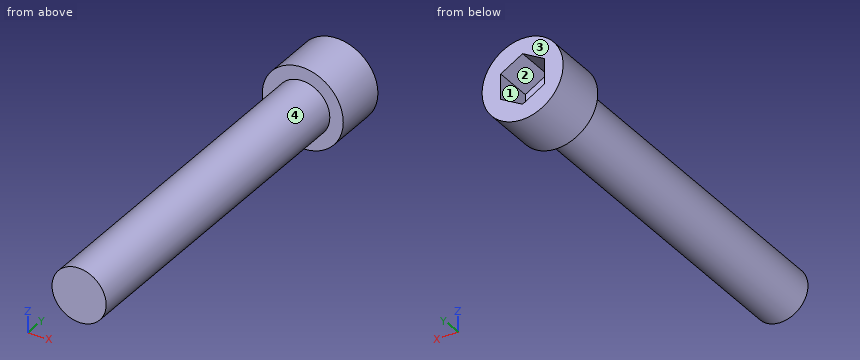
from build123d import *

# Parameters (mm, degrees)
SKETCH1_R           = 5.875
BOSS_EXTRUDE1_DEPTH = 7.75
CUT_EXTRUDE1_DEPTH  = 5.5
SKETCH3_R           = 3.925
BOSS_EXTRUDE2_DEPTH = 10
SKETCH4_R           = 3.925
BOSS_EXTRUDE3_DEPTH = 40


with BuildPart() as part:
    # Sketch1 → Boss-Extrude1 (new body)
    with BuildSketch(Plane(origin=(0, 0, 0), x_dir=(1, 0, 0), z_dir=(0, 1, 0))):
        Circle(SKETCH1_R)
    extrude(amount=BOSS_EXTRUDE1_DEPTH)

    # Sketch2 → Cut-Extrude1 (cut)
    with BuildSketch(Plane(origin=(0, 7.75, 0), x_dir=(1, 0, 0), z_dir=(0, 1, 0))):
        Polygon((0, 3.666174209), (-3.175, 1.833087105), (-3.175, -1.833087105), (0, -3.666174209), (3.175, -1.833087105), (3.175, 1.833087105), align=None)
    extrude(amount=-CUT_EXTRUDE1_DEPTH, mode=Mode.SUBTRACT)

    # Sketch3 → Boss-Extrude2 (add)
    with BuildSketch(Plane.XZ):
        Circle(SKETCH3_R)
    extrude(amount=BOSS_EXTRUDE2_DEPTH)

    # Sketch4 → Boss-Extrude3 (add)
    with BuildSketch(Plane.XZ.offset(10)):
        Circle(SKETCH4_R)
    extrude(amount=BOSS_EXTRUDE3_DEPTH)


solid = part.part
Check sheet for the modelled part. Datum: model origin and axes. Units: mm. Face numbers are marked on the shaded views. Give positions to 0.01 mm unless a question says otherwise; leave off trailing zeros. Loops run counter-clockwise (first coordinate to the right, second up) from the corner with the lowest first, then second, coordinate; pieces in that order, holes last. Notation, with made-up numbers: M -21.75,46 L 0.25,46 A30 cw 0.25,72 Z; hole C 44.25,37.5 d10. An arc over 180 degrees is marked long. Return JSON: item names as keys, results as strings. Group by question number.
1. Cross-section at C-C on y = -44. Record the boundary of the cut face in (x, z) (3 decimals).
2. Cross-section at B-B on x = 1.5. Record the boundary of the cut face in (y, z).
3. Thickness scan on L1, parallel to Y at x = -2.5, z = -4.5; L2, parallel to X at y = -5.5, z = -0.25; L3, parallel to Y at x = 2.5, z = 0.25. Record the ranges inside material, lowest first.
4. Mould release check, pull along Z, two halves, no side actions. Record for the marked faces 1, 2, 3 and 4: released by +Z, released by -Z, zero draft, split by the parting line, or undercut.
5. Cross-section at A-A on z = 0. Record the boundary of the cut face in (x, y) (3 decimals), plus the area to 3 significant figures.
6. Cross-section at D-D on z = -5. Record the boundary of the cut face in (x, y), plus the area to 3 significant figures.
7. Go/stop test with flat-tipped pins: pin 1 (5 mm diameter, centred on y = -19.5, z = -2.5, fed in from -X) (3 decimals); pin 2 (5 mm diameter, centred on x = 1.5, y = -29, fed in from -Z) (3 decimals); pin 3 (4 mm diameter, centred on y = -39, z = 4, fed in from -X). Record where each tip stops, or that it passes through.
Return value:
{
 "1": {"outline": "C 0,0 d7.85"},
 "2": {"outline": "M -50,-3.63 L 0,-3.63 L 0,-5.68 L 7.75,-5.68 L 7.75,-2.8 L 2.25,-2.8 L 2.25,2.8 L 7.75,2.8 L 7.75,5.68 L 0,5.68 L 0,3.63 L -50,3.63 Z"},
 "3": {"L1": "0 to 7.75", "L2": "-3.92 to 3.92", "L3": "-50 to 2.25"},
 "4": {"face 1": "undercut", "face 2": "undercut", "face 3": "zero draft", "face 4": "split by the parting line"},
 "5": {"outline": "M -5.875,0 L -3.925,0 L -3.925,-50 L 3.925,-50 L 3.925,0 L 5.875,0 L 5.875,7.75 L 3.175,7.75 L 3.175,2.25 L -3.175,2.25 L -3.175,7.75 L -5.875,7.75 Z", "area": "449 mm^2"},
 "6": {"outline": "M -3.08,0 L 3.08,0 L 3.08,7.75 L -3.08,7.75 Z", "area": "47.8 mm^2"},
 "7": {"pin 1": "x = -3.925", "pin 2": "z = -3.925", "pin 3": "x = -3.38"}
}
